Answer from the drawing. Dimensions are ordinates in mm from the lowest x, y and z of the part. Coordinates: 2 decimals unless noted, no trailing zeros. Answer as a JSON object with one key per item and string values. Group by question number.
(1) Straight lines are drawn through the part: L1, parallel to Z at x = 91.5, y = 2.25 (1 decimal); L2, parallel to Z at x = 55, y = 5.5 (1 decimal); L3, parallel to Y at x = 56, z = 20.25. For each, find the intervals that lie inside material, in ascending order.
(2) A flat-ended cylindrical pin translates along its axis: P1, Ø3, axis at x = 89.5, z = 10.5, coming from the +Y side. Find the tip coordinate at first contact, or state that the pin passes through.
(3) Find section A-A (z = 11). Count the separate pieces of the cut face and the enclosed holes in it, then the cut area to 3 significant figures.
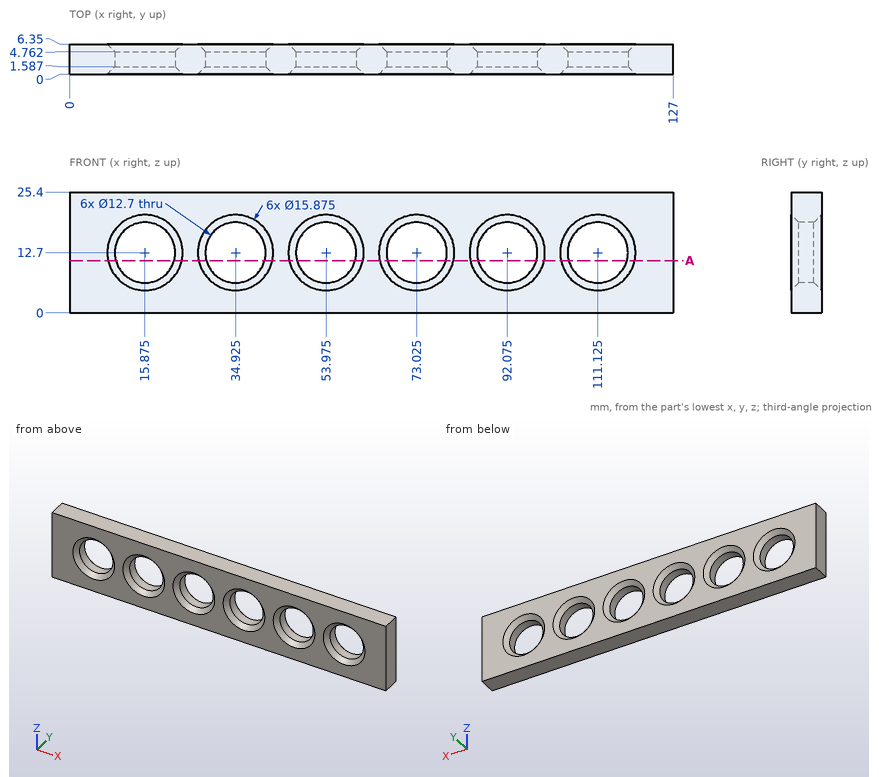
Results below:
{
 "1": {"L1": "z = 0 to 6.4, 19 to 25.4", "L2": "z = 0 to 5.7, 19.7 to 25.4", "L3": "y = 0.12 to 6.23"},
 "2": {"P1": "passes through"},
 "3": {"separate pieces": "7", "enclosed holes": "0", "area": "309 mm2"}
}
